For this review, use the dimensioned drawing (mm, ordinates from the lowest corner) and the shaded views. A direction names the side the tool comes from. Round coordinates to 2 decimals unless told otherwise and drop trailing zeros. Write each loop counter-clockwise with the first axis right and the second up, starting at its lowest first coordinate (ties: lowest second). Pieces come first, ordered by that corner, then holes. Notation, with made-up numbers: M 22,-28 L 41,-28 A26 ccw 41,8 Z; hole C 40,55 d8. An arc over 180 degrees is marked long. Use CSV: the item, a comma, the result in double quotes.
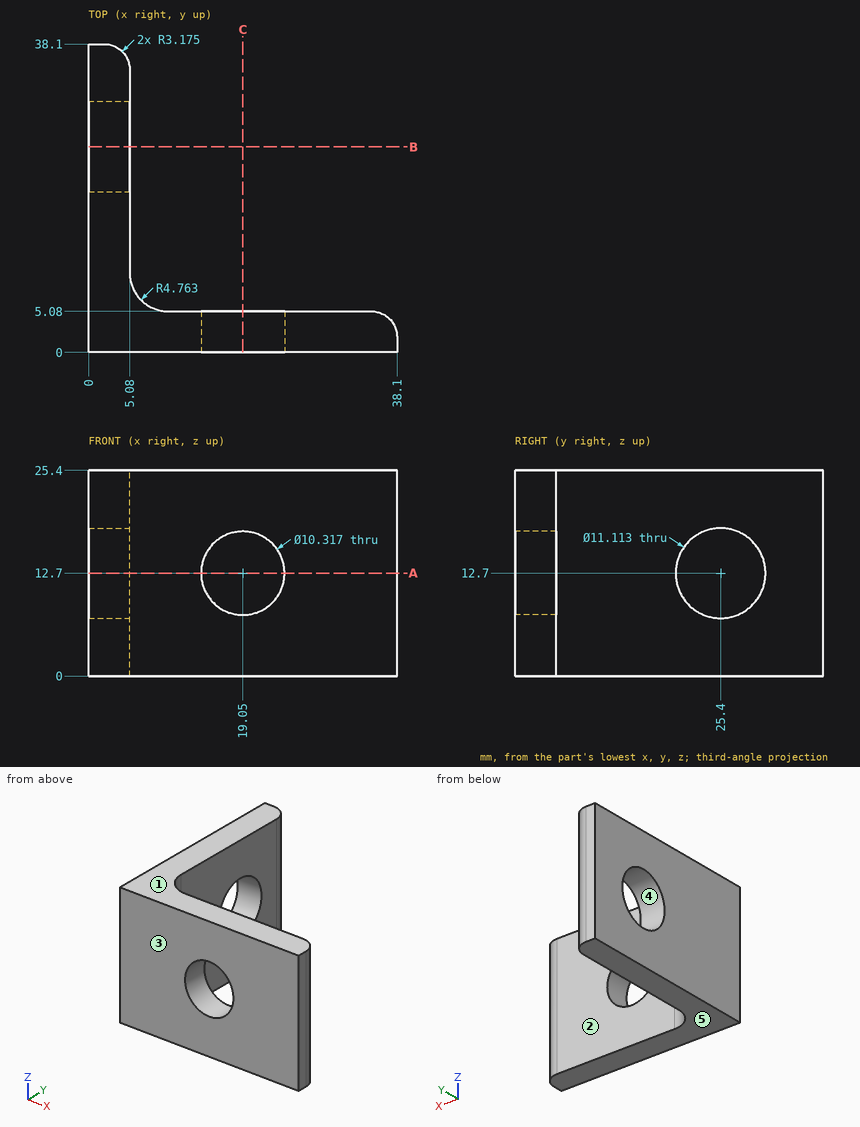
1) For pin 1 Ø13.5 at (x, z) = (19.05, 12.7) entering from +Y; pin 2 Ø6.5 at (y, z) = (25.4, 12.7) entering from +X, all flat-tipped, find the tip position at first contact; note any pin that passes through.
Answers:
pin 1,"y = 5.08"
pin 2,"through"
2) Add section B-B on y = 25.4. Write out the cut boundary in (x, z).
Answers:
outline,"M 0,0 L 5.08,0 L 5.08,7.14 L 0,7.14 Z; M 0,18.26 L 5.08,18.26 L 5.08,25.4 L 0,25.4 Z"
3) Add section C-C on x = 19.05. Write out the cut boundary in (y, z).
Answers:
outline,"M 0,0 L 5.08,0 L 5.08,7.54 L 0,7.54 Z; M 0,17.86 L 5.08,17.86 L 5.08,25.4 L 0,25.4 Z"
4) Wall thickness on line 1 along Z through (x, y) = (19.05, 1.65); line 2 along Y through (x, z) = (19, 19): over which ranges is each line inside the solid? List them lowest first. Write a range as [from, to].
Answers:
line 1,"[0, 7.54], [17.86, 25.4]"
line 2,"[0, 5.08]"
5) Machinability: for the marked faces 1 and 2, which of the approach directions +Z, -Z, +X, -X, +Y, -Y give a long, thin tool a straight path to every point of the face, cutting with its end or side? Answer none if there is none.
Answers:
face 1,"+Z, +X, -X, +Y, -Y"
face 2,"+Z, -Z, +X, +Y"
6) The part is to be moulded in two halves that separate along Y. For the marked faces 3, 4 and 5, say which applies: released by +Y, released by -Y, zero draft, split by the parting line, or undercut.
Answers:
face 3,"released by -Y"
face 4,"undercut"
face 5,"zero draft"
7) Add section A-A on z = 12.7. Give the number of separate pieces and of enclosed holes in the cut face, then the cut area to 3 significant figures.
Answers:
separate pieces,"3"
enclosed holes,"0"
area,"253 mm²"
